Autodesk Inventor part; units mm, degrees
ref_plane "YZ Plane" through (0, 0, 0) normal (1, 0, 0) x (0, 1, 0)
ref_plane "XZ Plane" through (0, 0, 0) normal (0, 1, 0) x (-1, 0, 0)
ref_plane "XY Plane" through (0, 0, 0) normal (0, 0, 1) x (1, 0, 0)
sketch "Sketch1" plane through (0, 0, 0) normal (0, 1, 0) x (-1, 0, 0)
  circle A0 centre (0, 0) radius 425
  circle A1 centre (0, 0) radius 233.71
  dimension "d84" = 467.42
  dimension "d85" = 850
extrude "Extrusion3" add sketch "Sketch1" along normal blind 6
sketch "Sketch2" plane through (0, 6, 0) normal (0, 1, 0) x (1, 0, 0)
  circle A0 centre (0, 0) radius 329.355 construction
  line L0 (3.25, 363.0217) -> (3.25, 295.6883)
  line L1 (-3.25, 295.6883) -> (-3.25, 363.0217)
  arc A1 (-3.25, 295.6883) -> (-1.9167, 294.355) centre (-1.9167, 295.6883) ccw
  arc A2 (1.9167, 294.355) -> (3.25, 295.6883) centre (1.9167, 295.6883) ccw
  arc A3 (-1.9167, 364.355) -> (-3.25, 363.0217) centre (-1.9167, 363.0217) ccw
  arc A4 (3.25, 363.0217) -> (1.9167, 364.355) centre (1.9167, 363.0217) ccw
  line L2 (-1.9167, 364.355) -> (1.9167, 364.355)
  line L3 (-1.9167, 294.355) -> (1.9167, 294.355)
  line L4 (0, 294.355) -> (0, 329.355) construction
  line L5 (0, 364.355) -> (0, 329.355) construction
  line L6 (0, 364.355) -> (0, 294.355) construction
  line L7 (175.0629, -238.5433) -> (171.9617, -240.7965)
  arc A5 (176.9253, -238.8383) -> (175.0629, -238.5433) centre (175.8467, -239.622) ccw
  arc A6 (171.9617, -240.7965) -> (171.6667, -242.6589) centre (172.7454, -241.8752) ccw
  line L8 (173.0175, -238.1382) -> (193.59, -266.4538) construction
  line L9 (211.2443, -297.1327) -> (171.6667, -242.6589)
  line L10 (176.9253, -238.8383) -> (216.5029, -293.3121)
  line L11 (214.1625, -294.7694) -> (173.0175, -238.1382) construction
  line L12 (214.1625, -294.7694) -> (193.59, -266.4538) construction
  arc A7 (211.2443, -297.1327) -> (213.1067, -297.4277) centre (212.323, -296.349) ccw
  line L13 (216.2079, -295.1745) -> (213.1067, -297.4277)
  arc A8 (216.2079, -295.1745) -> (216.5029, -293.3121) centre (215.4242, -294.0958) ccw
  line L14 (280.1548, 92.2019) -> (281.3393, 88.5562)
  arc A9 (281.0108, 93.882) -> (280.1548, 92.2019) centre (281.4229, 92.614) ccw
  arc A10 (281.3393, 88.5562) -> (283.0194, 87.7002) centre (282.6074, 88.9682) ccw
  line L15 (279.9482, 90.9607) -> (313.2352, 101.7763) construction
  line L16 (347.0573, 108.5073) -> (283.0194, 87.7002)
  line L17 (281.0108, 93.882) -> (345.0486, 114.6892)
  line L18 (346.5222, 112.5919) -> (279.9482, 90.9607) construction
  line L19 (346.5222, 112.5919) -> (313.2352, 101.7763) construction
  arc A11 (347.0573, 108.5073) -> (347.9133, 110.1874) centre (346.6452, 109.7754) ccw
  line L20 (346.7287, 113.8331) -> (347.9133, 110.1874)
  arc A12 (346.7287, 113.8331) -> (345.0486, 114.6892) centre (345.4607, 113.4211) ccw
  dimension "d86" = 658.71
  dimension "d21" = 6.5
  dimension "d24" = 2.6667
  dimension "d25" = 2.6667
  dimension "d32" = 1.3333
  dimension "d33" = 1.3333
  dimension "d162" = 70
  dimension "d163" = 294.355
  dimension "d165" = 3.25
extrude "Extrusion4" cut sketch "Sketch2" against normal through all
sketch "Sketch3" plane through (0, 6, 0) normal (0, 1, 0) x (1, 0, 0)
  arc A0 (-131.3389, -404.1968) -> (131.3445, -404.195) centre (0, 0) ccw
  arc A1 (-77.7244, -128.3741) -> (77.7297, -128.3709) centre (0, 0) ccw
  line L0 (-122.1811, -173.696) -> (-161.3589, -227.6196)
  line L1 (-131.3389, -404.1968) -> (-77.7244, -128.3741)
  line L2 (0, 0) -> (0, -341.2918)
  line L3 (131.3445, -404.195) -> (77.7297, -128.3709)
  line L4 (210.5535, -295.3313) -> (171.3679, -241.3969)
  dimension "d52" = 25
  dimension "d87" = 150.07
  dimension "d88" = 425
  dimension "d89" = 25
  dimension "d90" = 11
  dimension "d91" = 11
sketch "Sketch5" plane through (0, 6, 0) normal (0, 1, 0) x (1, 0, 0)
  line L0 (3.25, 363.0217) -> (3.25, 295.6883)
  line L1 (5.5862, 281.6788) -> (-6.155, 278.5328)
  line L2 (-11.2263, 385.43) -> (10.5847, 377.0575)
  line L3 (6.5657, 233.6709) -> (8.9394, 278.9635)
  line L4 (14.2034, 379.4075) -> (16.5771, 424.7001)
  arc A0 (10.5847, 377.0575) -> (14.2034, 379.4075) centre (11.5404, 379.5471) ccw
  arc A1 (8.9394, 278.9635) -> (5.5862, 281.6788) centre (6.2763, 279.103) ccw
  arc A2 (-11.2263, 385.43) -> (-14.8449, 382.8009) centre (-12.1819, 382.9405) ccw
  line L5 (-3.25, 295.6883) -> (-3.25, 363.0217)
  line L6 (-14.8449, 382.8009) -> (-9.5081, 280.969)
  arc A3 (-9.5081, 280.969) -> (-6.155, 278.5328) centre (-6.8451, 281.1086) ccw
  line L7 (-1.9167, 294.355) -> (1.9167, 294.355)
  line L8 (1.9167, 364.355) -> (-1.9167, 364.355)
  line L9 (16.5771, 424.7001) -> (16.5774, 424.7058)
  line L10 (6.5657, 233.6709) -> (6.5621, 233.6028)
  circle A4 centre (0, 0) radius 425
  circle A5 centre (0, 0) radius 233.71
  line L11 (-356.4489, 130.7516) -> (-398.7912, 147.0053)
  arc A6 (-355.3322, 126.5839) -> (-356.4489, 130.7516) centre (-357.4046, 128.2621) ccw
  line L12 (-370.0348, 108.4276) -> (-355.3322, 126.5839)
  arc A7 (-370.0348, 108.4276) -> (-368.6526, 104.1736) centre (-367.9624, 106.7494) ccw
  line L13 (-368.6526, 104.1736) -> (-270.1556, 77.7814)
  arc A8 (-270.1556, 77.7814) -> (-266.8024, 80.2177) centre (-269.4654, 80.3572) ccw
  line L14 (-266.1663, 92.3563) -> (-266.8024, 80.2177)
  arc A9 (-262.5476, 94.7063) -> (-266.1663, 92.3563) centre (-263.5032, 92.2167) ccw
  line L15 (-220.2053, 78.4526) -> (-262.5476, 94.7063)
  line L16 (-220.2053, 78.4526) -> (-220.1417, 78.4282)
  line L17 (-398.7912, 147.0053) -> (-398.7965, 147.0073)
  line L18 (-142.66, -185.1845) -> (-142.6172, -185.1316)
  line L19 (-263.0436, -333.8458) -> (-263.0472, -333.8502)
  line L20 (132.0366, -192.9029) -> (131.9995, -192.8458)
  line L21 (236.2213, -353.3334) -> (236.2244, -353.3381)
  line L22 (365.2271, 103.7351) -> (409.0364, 115.4738)
  arc A10 (361.8739, 106.4505) -> (365.2271, 103.7351) centre (364.5369, 106.3109) ccw
  line L23 (363.0966, 129.7812) -> (361.8739, 106.4505)
  arc A11 (363.0966, 129.7812) -> (359.478, 132.4103) centre (360.4336, 129.9208) ccw
  line L24 (359.478, 132.4103) -> (264.2793, 95.867)
  arc A12 (264.2793, 95.867) -> (262.9985, 91.9251) centre (265.2349, 93.3774) ccw
  line L25 (269.6187, 81.7308) -> (262.9985, 91.9251)
  arc A13 (268.0724, 77.7026) -> (269.6187, 81.7308) centre (267.3822, 80.2784) ccw
  line L26 (224.2631, 65.9639) -> (268.0724, 77.7026)
  line L27 (224.2631, 65.9639) -> (224.1973, 65.9463)
  line L28 (409.0364, 115.4738) -> (409.0419, 115.4753)
  line L29 (0, -233.71) -> (0, -425)
  arc A14 (131.3445, -404.195) -> (-131.3389, -404.1968) centre (0, 0) ccw
  point P0 (-425, 0)
  point P1 (-425, 0)
  point P2 (-398.7693, 146.9969)
  point P3 (-220.1557, 78.4336)
  point P4 (16.5759, 424.6766)
  point P5 (6.5629, 233.6178)
  point P6 (409.0137, 115.4677)
  point P7 (224.2118, 65.9502)
  dimension "d63" = 2.6667
  dimension "d64" = 3
  dimension "d66" = 3
  dimension "d67" = 2.6667
  dimension "d68" = 2.6667
  dimension "d70" = 72
  dimension "d71" = 72
sketch "Sketch6" plane through (0, 6, 0) normal (0, 1, 0) x (1, 0, 0)
  line L0 (237.9351, -331.8846) -> (247.6433, -324.8312)
  line L1 (243.8227, -319.5725) -> (234.1145, -326.626)
  line L2 (210.5535, -295.3313) -> (171.3679, -241.3969)
  line L3 (215.5172, -293.3731) -> (212.416, -295.6263)
  arc A0 (244.7539, -319.72) -> (243.8227, -319.5725) centre (244.2145, -320.1119) ccw
  arc A1 (247.6433, -324.8312) -> (247.7908, -323.9) centre (247.2514, -324.2918) ccw
  arc A2 (237.0039, -331.7371) -> (237.9351, -331.8846) centre (237.5432, -331.3452) ccw
  arc A3 (234.1145, -326.626) -> (233.967, -327.5572) centre (234.5063, -327.1653) ccw
  line L4 (233.967, -327.5572) -> (237.0039, -331.7371)
  line L5 (247.7908, -323.9) -> (244.7539, -319.72)
  line L6 (171.3679, -241.3969) -> (210.5535, -295.3313)
  line L7 (190.9607, -268.3641) -> (196.2193, -264.5435)
  line L8 (215.8122, -291.5107) -> (176.6265, -237.5763)
  line L9 (145.065, -204.0599) -> (154.7732, -197.0065)
  line L10 (158.5938, -202.2651) -> (148.8856, -209.3185)
  arc A4 (158.5938, -202.2651) -> (158.7413, -201.3339) centre (158.202, -201.7257) ccw
  arc A5 (155.7044, -197.154) -> (154.7732, -197.0065) centre (155.1651, -197.5458) ccw
  arc A6 (145.065, -204.0599) -> (144.9175, -204.9911) centre (145.4569, -204.5992) ccw
  arc A7 (147.9544, -209.171) -> (148.8856, -209.3185) centre (148.4938, -208.7792) ccw
  line L11 (147.9544, -209.171) -> (144.9175, -204.9911)
  line L12 (155.7044, -197.154) -> (158.7413, -201.3339)
  point P0 (0, 0)
  dimension "d104" = 6.5
  dimension "d105" = 12
  dimension "d108" = 1.3333
  dimension "d109" = 1.3333
  dimension "d110" = 1.3333
  dimension "d111" = 1.3333
  dimension "d112" = 0
  dimension "d149" = 145
  dimension "d150" = 90
  dimension "d151" = 90
  dimension "d152" = 90
  dimension "d153" = 90
extrude "Extrusion7" cut sketch "Sketch6" against normal through all
pattern_circular "Circular Pattern2" count 2 over 72 about axis through (0, -10, 0) along (0, 1, 0) of "Extrusion7"
pattern_circular "Circular Pattern3" count 2 over 144 about axis through (0, -10, 0) along (0, 1, 0) of "Extrusion7"
mirror "Mirror3" about plane through (0, 0, 0) normal (1, 0, 0) of "Extrusion7"
extrude "Extrusion10" cut sketch "Sketch3" against normal blind 10
mirror "Mirror4" about plane through (0, 0, 0) normal (1, 0, 0) of "Extrusion4"
pattern_circular "Circular Pattern4" count 2 over 144 about axis through (0, -10, 0) along (0, -1, 0) of "Extrusion7"
extrude "Extrusion11" cut sketch "Sketch5" against normal through all contours A1 L3 L10 A5 L16 L15 A9 L14 A8 L13 A7 L12 A6 L11 A4 L4 A0 L2 A2 L6 A3 L1 | L1 A3 L6 A2 L2 A0 L4 A4 L22 A10 L23 A11 L24 A12 L25 A13 L26 L27 A5 L10 L3 A1 | A5 L29 A4 L11 A6 L12 A7 L13 A8 L14 A9 L15 L16
equation "\"BendRadius\" = Thickness"
equation "\"BendReliefWidth\" = Thickness"
equation "\"BendReliefDepth\" = 0.5 * Thickness"
equation "\"CornerReliefSize\" = 4 * Thickness"
equation "\"MinimumRemnant\" = 2 * Thickness"
equation "\"TransitionRadius\" = BendRadius"
equation "\"JacobiRadiusSize\" = BendRadius"
equation "\"GapSize\" = Thickness"
properties part number "Ring C4" material "Wood (Maple)"
Part model, mm, in its own coordinate system. A direction names the side the tool comes from. Give positions to 0.01 mm unless a question says otherwise; leave off trailing zeros. Loops run counter-clockwise (first coordinate to the right, second up) from the corner with the lowest first, then second, coordinate; pieces in that order, holes last.
(1) Band-saw the part on D-D (x = 118). Write the cut outline in (y, z), and give its area (3 significant figures).
Return value:
outline: (0, 201.73) - (6, 201.73) - (6, 335.54) - (0, 335.54) - close
area: 803 mm2
(2) Band-saw the part on A-A (x = 318). Write the cut outline in (y, z), and give its area (3 significant figures).
Return value:
outline: (0, -116.49) - (6, -116.49) - (6, -105.9) - (0, -105.9) - close; (0, -99.07) - (6, -99.07) - (6, 281.96) - (0, 281.96) - close
area: 2,350 mm2
(3) Pin check, flat tips, straight feed: pin 1 (1.5 mm diameter, centred on x = 358, y = 2.5, fed in from +Z); pin 2 (1.5 mm diameter, centred on x = 292, y = 2.5, fed in from +Z); pin 3 (3 mm diameter, centred on y = 5, z = 294, fed in from -X). Stop position of each tip, or through.
Return value:
pin 1: stops at z = 230.21
pin 2: stops at z = 309.51
pin 3: stops at x = 109.63
(4) Band-saw the part on C-C (y = 1.75). Count the separate pieces of the cut face and the enclosed holes in it, and give its area (3 significant figures).
Return value:
separate pieces: 1
enclosed holes: 4
area: 95,800 mm2
(5) Drill centre lines: line 1 along Z through (x, y) = (212, 5.65); line 2 along Z through (x, y) = (236, 5.3); line 3 along X through (y, z) = (5.5, 88.5). Where is each one in solid material? Low to high.
Return value:
line 1: z = 98.37 to 287.11, 297.64 to 368.35
line 2: z = -69.11 to 325.26, 330.36 to 353.45
line 3: x = 216.31 to 415.68
(6) 3-axis set-ups, long thin cutter, end or side, ignore diameter. For faces 4 (the flat face through (191.733, 3.042, 270.277)), 5 (the flat face through (386.81, 3.04, -109.52)), 6 (the cylindrical face through (212.966, 2.958, 96.26)): which of +Z, -Z, +X, -X, +Y, -Y reach the whole face in a straight line?
Return value:
face 4: +Y, -Y
face 5: -Z, +Y, -Y
face 6: -X, +Y, -Y
(7) Pull direction Z, two halves, no side cores. Call faces 1 (the flat face through (312.58, 3.04, -104.14)), 2 (the flat face through (299, 0, 140)), 3 (the cylindrical face through (376.97, 2.96, 196.26)): pulls with the +Z half, pulls with the -Z half, needs draft (parallel to the pull), parting line crosses it, or undercut.
Return value:
face 1: undercut
face 2: needs draft
face 3: parting line crosses it
(8) Band-saw the part on B-B (z = 272). Write the cut outline in (x, y), and give its area (3 significant figures).
Return value:
outline: (105.65, 0) - (192.98, 0) - (192.98, 6) - (105.65, 6) - close; (201.02, 0) - (326.56, 0) - (326.56, 6) - (201.02, 6) - close
area: 1,280 mm2
